Source: CAD feature listing. Evaluate the final solid. Frame: model axes, mm. A direction names the side the tool comes from. Give positions to 0.01 mm unless a question says otherwise; leave off trailing zeros. Write each loop counter-clockwise with the first axis right and the second up, starting at its lowest first coordinate (ties: lowest second). Pieces come first, ordered by that corner, then holes. Notation, with made-up numbers: (36.25, -32) -> (54.25, -32) arc R13 ccw to (54.25, -15) -> close; hole circle Ø3 at (-33, -23.75). An arc over 180 degrees is marked (long way). Write item = value, one per line.
from build123d import *

# Parameters (mm, degrees)
ESQUISSE2_R                  = 10
ENL_V_MAT_EXTRU_1_DEPTH      = 687.62944883
R_P_TITION_CIRCULAIRE1_COUNT = 20
BOSS_EXTRU_1_START           = -10
ESQUISSE5_R                  = 436
ESQUISSE5_R_2                = 336
BOSS_EXTRU_1_DEPTH           = 10
BOSS_EXTRU_2_START           = 115
ESQUISSE6_R                  = 436
ESQUISSE6_R_2                = 426
BOSS_EXTRU_2_DEPTH           = 115
BOSS_EXTRU_3_START           = -10
BOSS_EXTRU_3_DEPTH           = 10
BOSS_EXTRU_4_START           = 115
BOSS_EXTRU_4_DEPTH           = 115
ENL_V_MAT_EXTRU_3_DEPTH      = 115
R_P_TITION_CIRCULAIRE6_COUNT = 2
ESQUISSE10_R                 = 336
ENL_V_MAT_EXTRU_4_DEPTH      = 80


with BuildPart() as part:
    # Esquisse1 → Révolution1 (revolve)
    with BuildSketch(Plane.XY, mode=Mode.PRIVATE) as r_volution1_sk:
        with BuildLine():
            Line((0, 0), (80, 0))
            Line((80, 0), (80, 52.5))
            ThreePointArc((80, 52.5), (70, 62.5), (80, 72.5))
            Line((80, 72.5), (80, 90))
            Line((80, 90), (0, 90))
            Line((0, 90), (0, 0))
        make_face()
    revolve(r_volution1_sk.sketch.rotate(Axis((-256, 27.419354839, 0), (0, -1, 0)), 90), axis=Axis((-256, 27.419354839, 0), (0, -1, 0)))

    # Esquisse2 → Enlèv. mat.-Extru.1 (cut, through all)
    with BuildSketch(Plane.XZ):
        with Locations(Location((40, 0, 0), (0, 0, 270))):
            Circle(ESQUISSE2_R)
    enl_v_mat_extru_1 = extrude(amount=-ENL_V_MAT_EXTRU_1_DEPTH, mode=Mode.SUBTRACT)

    # Répétition circulaire1: Enlèv. mat.-Extru.1 ×20 about axis
    r_p_tition_circulaire1_axis = Axis((-256, 0, 0), (0, 1, 0))
    for i in range(1, R_P_TITION_CIRCULAIRE1_COUNT):
        add(enl_v_mat_extru_1.rotate(r_p_tition_circulaire1_axis, i * 360 / R_P_TITION_CIRCULAIRE1_COUNT), mode=Mode.SUBTRACT)

    # Esquisse5 → Boss.-Extru.1 (add)
    with BuildSketch(Plane.XZ.offset(BOSS_EXTRU_1_START)):
        with Locations(Location((-256, 0, 0), (0, 0, 270))):
            Circle(ESQUISSE5_R)
        with Locations(Location((-256, 0, 0), (0, 0, 90))):
            Circle(ESQUISSE5_R_2, mode=Mode.SUBTRACT)
    extrude(amount=BOSS_EXTRU_1_DEPTH)

    # Esquisse6 → Boss.-Extru.2 (add)
    with BuildSketch(Plane(origin=(0, 10, 0), x_dir=(1, 0, 0), z_dir=(0, 1, 0)).offset(BOSS_EXTRU_2_START)):
        with Locations(Location((-256, 0, 0), (0, 0, 90))):
            Circle(ESQUISSE6_R)
        with Locations(Location((-256, 0, 0), (0, 0, 270))):
            Circle(ESQUISSE6_R_2, mode=Mode.SUBTRACT)
    extrude(amount=-BOSS_EXTRU_2_DEPTH)

    # Esquisse7 → Boss.-Extru.3 (add)
    with BuildSketch(Plane.XZ.offset(BOSS_EXTRU_3_START)):
        with BuildLine():
            Line((93.994285668, 260), (263.994285668, 260))
            Line((263.994285668, 260), (263.994285668, -260))
            Line((263.994285668, -260), (93.994285668, -260))
            ThreePointArc((93.994285668, -260), (180, 0), (93.994285668, 260))
        make_face()
    boss_extru_3 = extrude(amount=BOSS_EXTRU_3_DEPTH)

    # Esquisse8 → Boss.-Extru.4 (add)
    with BuildSketch(Plane(origin=(0, 10, 0), x_dir=(1, 0, 0), z_dir=(0, 1, 0)).offset(BOSS_EXTRU_4_START)):
        with BuildLine():
            Line((113.345366832, 250), (253.994285668, 250))
            Line((253.994285668, 250), (253.994285668, -250))
            Line((253.994285668, -250), (113.345366832, -250))
            Line((113.345366832, -250), (101.205823021, -250))
            ThreePointArc((101.205823021, -250), (97.635403251, -255.025491996), (93.994285668, -260))
            Line((93.994285668, -260), (263.994285668, -260))
            Line((263.994285668, -260), (263.994285668, 260))
            Line((263.994285668, 260), (93.994285668, 260))
            ThreePointArc((93.994285668, 260), (97.635403251, 255.025491996), (101.205823021, 250))
            Line((101.205823021, 250), (113.345366832, 250))
        make_face()
    boss_extru_4 = extrude(amount=-BOSS_EXTRU_4_DEPTH)

    # Esquisse9 → Enlèv. mat.-Extru.3 (cut)
    with BuildSketch(Plane(origin=(0, 125, 0), x_dir=(1, 0, 0), z_dir=(0, 1, 0))):
        with BuildLine():
            Line((101.205823021, -250), (88.928978197, -250))
            ThreePointArc((88.928978197, -250), (170, 0), (88.928978197, 250))
            Line((88.928978197, 250), (101.205823021, 250))
            ThreePointArc((101.205823021, 250), (180, 0), (101.205823021, -250))
        make_face()
    enl_v_mat_extru_3 = extrude(amount=-ENL_V_MAT_EXTRU_3_DEPTH, mode=Mode.SUBTRACT)

    # Répétition circulaire6: Boss.-Extru.3, Boss.-Extru.4, Enlèv. mat.-Extru.3 ×2 about axis
    r_p_tition_circulaire6_axis = Axis((-256, 0, 0), (0, 1, 0))
    add([boss_extru_3.rotate(r_p_tition_circulaire6_axis, i * 360 / R_P_TITION_CIRCULAIRE6_COUNT) for i in range(1, R_P_TITION_CIRCULAIRE6_COUNT)])
    add([boss_extru_4.rotate(r_p_tition_circulaire6_axis, i * 360 / R_P_TITION_CIRCULAIRE6_COUNT) for i in range(1, R_P_TITION_CIRCULAIRE6_COUNT)])
    add([enl_v_mat_extru_3.rotate(r_p_tition_circulaire6_axis, i * 360 / R_P_TITION_CIRCULAIRE6_COUNT) for i in range(1, R_P_TITION_CIRCULAIRE6_COUNT)], mode=Mode.SUBTRACT)

    # Esquisse10 → Enlèv. mat.-Extru.4 (cut)
    with BuildSketch(Plane(origin=(0, 90, 0), x_dir=(1, 0, 0), z_dir=(0, 1, 0))):
        with Locations((-256, 0)):
            Circle(ESQUISSE10_R)
    extrude(amount=-ENL_V_MAT_EXTRU_4_DEPTH, mode=Mode.SUBTRACT)


solid = part.part
(1) First-contact query: pin 1 (8 mm diameter, centred on y = 101.5, z = 305, fed in from +X); pin 2 (1 mm diameter, centred on x = -461, y = 13, fed in from +Z); pin 3 (16 mm diameter, centred on x = -429.98, z = 239.47, fed in from -Y); pin 4 (6 mm diameter, centred on x = -343, y = 97, fed in from +Z). Flat tips, straight axial feed; report the tip coordinate or a pass-through.
Values follow:
pin_1 = 59.43
pin_2 = 385.07
pin_3 = through
pin_4 = 427.83
(2) Material intervals for line 1 (X direction, y = 7.5, z = 0); line 2 (X direction, y = 16, z = 1); line 3 (Z direction, x = -620.5, y = 53), sorted ascending.
Values follow:
line_1 = -775.99 to -562, -542 to -512, 0 to 30, 50 to 263.99
line_2 = -775.99 to -765.99, 253.99 to 263.99
line_3 = -260 to -250, 250 to 260
(3) Section query A-A (y = 38). Return loops of the section in (x, z), plus the area to 3 significant figures.
Values follow:
outline = (-775.99, -260) -> (-605.99, -260) arc R436 ccw to (93.99, -260) -> (263.99, -260) -> (263.99, 260) -> (93.99, 260) arc R436 ccw to (-605.99, 260) -> (-775.99, 260) -> close; hole (-765.99, -250) -> (-600.93, -250) arc R426 ccw to (88.93, -250) -> (253.99, -250) -> (253.99, 250) -> (88.93, 250) arc R426 ccw to (-600.93, 250) -> (-765.99, 250) -> close
area = 33,100 mm2
(4) Access query for faces 1 (the face through (180, 63, -260)), 2 (the face through (-690, 63, -260)), 3 (the face through (178, 63, 260)), 4 (the face through (253.994, 68, -3)), 5 (the face through (-692, 63, 260)). Directions: +Z, -Z, +X, -X, +Y, -Y. A direction counts if a zero-diameter tool reaches every point of the face in a straight line with its end or side. Return the directions, or none.
Values follow:
face_1 = -Z, +X, +Y, -Y
face_2 = -Z, -X, +Y, -Y
face_3 = +Z, +X, +Y, -Y
face_4 = +Y
face_5 = +Z, -X, +Y, -Y
(5) Section query C-C (z = -43). Return loops of the section in (x, y), plus the area to 3 significant figures.
Values follow:
outline = (-775.99, 0) -> (-508.36, 0) -> (-508.36, 10) -> (-765.99, 10) -> (-765.99, 125) -> (-775.99, 125) -> close; (-3.64, 0) -> (263.99, 0) -> (263.99, 125) -> (253.99, 125) -> (253.99, 10) -> (-3.64, 10) -> close
area = 7,650 mm2
(6) Section query B-B (x = -122.5). Return loops of the section in (y, z).
Values follow:
outline = (0, -415.06) -> (125, -415.06) -> (125, -404.54) -> (10, -404.54) -> (10, -218.43) -> (0, -218.43) -> close; (0, 218.43) -> (10, 218.43) -> (10, 404.54) -> (125, 404.54) -> (125, 415.06) -> (0, 415.06) -> close
(7) Pull-direction query (X, two-part tool) for faces 6 (the face through (263.994, 63, 4)), 7 (the face through (-61, 125, -386)), 8 (the face through (-775.994, 63, -4)), 9 (the face through (-765.994, 68, 3)); classes: pulls with the +X half, pulls with the -X half, needs draft (parallel to the pull), parting line crosses it, or undercut.
Values follow:
face_6 = pulls with the +X half
face_7 = needs draft
face_8 = pulls with the -X half
face_9 = undercut
(8) Section query D-D (z = -372). Return loops of the section in (x, y), plus the area to 3 significant figures.
Values follow:
outline = (-483.4, 0) -> (-28.6, 0) -> (-28.6, 125) -> (-48.41, 125) -> (-48.41, 10) -> (-463.59, 10) -> (-463.59, 125) -> (-483.4, 125) -> close
area = 9,110 mm2
